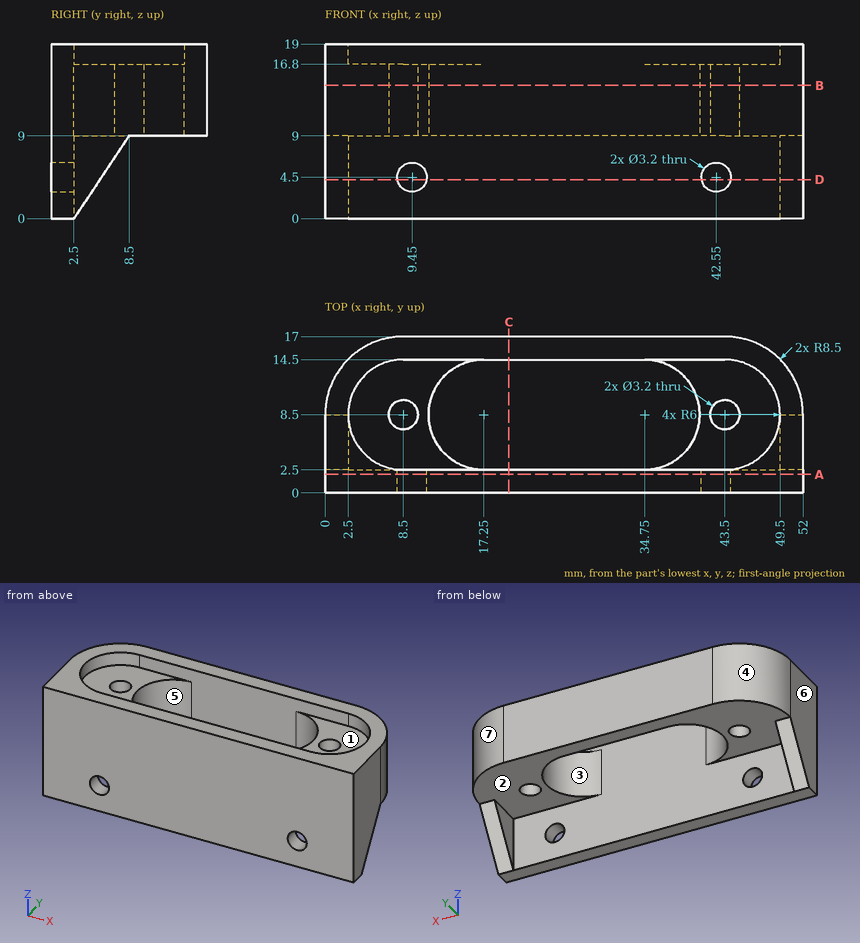
Could you check a few things on this drawing? It's one solid part, dimensions in mm from its lowest x, y, z. A direction names the side the tool comes from. Give positions to 0.01 mm unless a question says otherwise; leave off trailing zeros. Order: outer loops, then holes, each group sorted by start corner. A loop starts at its lowest first (then second) coordinate and runs counter-clockwise, first axis right, second up. Notation, with made-up numbers: M -22.75,9.25 L 35.25,9.25 A19 cw 35.25,32.25 Z; hole C -1,9.25 d3. An arc over 180 degrees is marked long. Use one line per item in the form item = value. Start each with the question number.
Item 1: For the marked faces 1, 2, 3 and 4, which set-ups out of +Z, -Z, +X, -X, +Y, -Y let a thin tool reach every point of the face, with its end or its side?
Item 2: If we section it at A-A (y = 2): Write out the boundary of the cut face in (x, z), then the cut area to 3 significant figures.
Item 3: If we section it at C-C (x = 20): Write out the boundary of the cut face in (y, z), then the cut area to 3 significant figures.
Item 4: Will these pins go through, and if not, where does the flat tip stop? pin 1 Ø5 at (x, y) = (8.5, 8.5) entering from -Z; pin 2 Ø3.5 at (x, z) = (9.45, 4.5) entering from +Y; pin 3 Ø3.5 at (x, y) = (41, 6) entering from +Z.
Item 5: If I drill on line 1 along Y through (x, z) = (15, 18); line 2 along Y through (x, z) = (15, 8.75); line 3 along X through (y, z) = (12.5, 14), over which ranges is the centre line in solid material (lowest first)?
Item 6: If we section it at B-B (z = 14.5): Write out the boundary of the cut face in (x, y), then the cut area to 3 significant figures.
Item 7: We'd pull the mould along Y, two halves only. Please class the marked faces 5, 6 and 7: +Y half, -Y half, draft (parallel to the pull), parting line (faces both ways), or undercut.
Item 8: If we section it at D-D (z = 4.25): Write out the boundary of the cut face in (x, y).
Outcome:
q1.face_1 = +Z
q1.face_2 = -Z, +Y
q1.face_3 = +Z, -Z
q1.face_4 = +Z, -Z, -X, +Y
q2.outline = M 0,0 L 52,0 L 52,19 L 0,19 Z; hole C 9.45,4.5 d3.2; hole C 42.55,4.5 d3.2
q2.area = 972 mm2
q3.outline = M 0,0 L 2.5,0 L 2.5,19 L 0,19 Z; M 14.5,9 L 17,9 L 17,19 L 14.5,19 Z
q3.area = 72.5 mm2
q4.pin_1 = 9
q4.pin_2 = 2.5
q4.pin_3 = 16.8
q5.line_1 = 0 to 2.5, 14.5 to 17
q5.line_2 = 0 to 2.5
q5.line_3 = 1 to 12.78, 39.22 to 51
q6.outline = M 0,0 L 52,0 L 52,8.5 A8.5 ccw 43.5,17 L 8.5,17 A8.5 ccw 0,8.5 Z; hole C 8.5,8.5 d3.2; hole M 17.25,2.5 L 34.75,2.5 A6 ccw 34.75,14.5 L 17.25,14.5 A6 ccw Z; hole C 43.5,8.5 d3.2
q6.area = 514 mm2
q7.face_5 = undercut
q7.face_6 = draft
q7.face_7 = +Y half
q8.outline = M 0,0 L 7.87,0 L 7.87,2.5 L 2.5,2.5 L 2.5,5.33 L 0,5.33 Z; M 11.03,0 L 40.97,0 L 40.97,2.5 L 11.03,2.5 Z; M 44.13,0 L 52,0 L 52,5.33 L 49.5,5.33 L 49.5,2.5 L 44.13,2.5 Z
